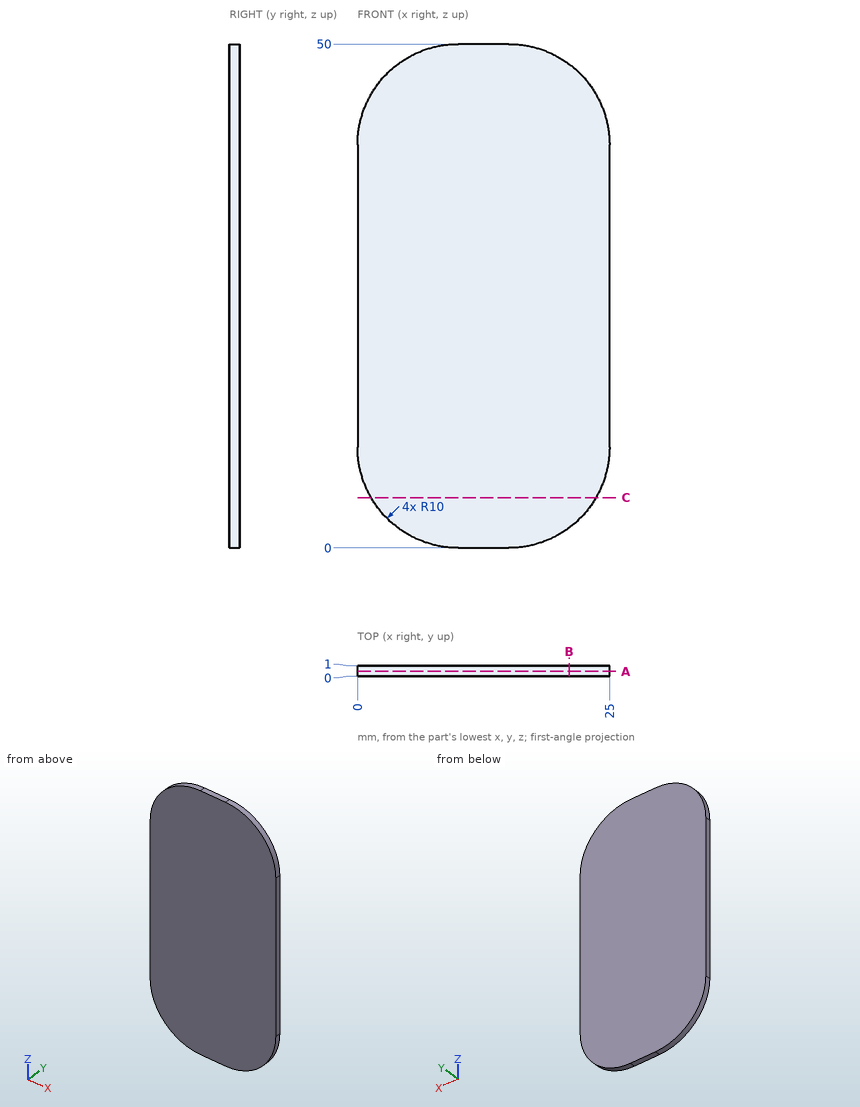
Verification items for this drawing (mm, ordinates from the low corner). Coordinates: 2 decimals unless noted, no trailing zeros. Order: outer loops, then holes, each group sorted by start corner. A loop starts at its lowest first (then second) coordinate and runs counter-clockwise, first axis right, second up. Notation, with made-up numbers: (88.25, 9.5) - (144.25, 9.5) arc R34 cw to (144.25, 43.5) - close; hole circle Ø3 at (63, 32.25). An arc over 180 degrees is marked (long way). Answer in a Markdown table with one row per item. Add a question column.
1. Section check B-B (x = 21). Enter the section's corners in (y, z), plus the area to 3 significant figures.
2. Section check C-C (z = 5). Enter the section's corners in (x, y), plus the area to 3 significant figures.
3. Section check A-A (y = 0.45). Enter the section's corners in (x, z).
4. Material ranges on L1, parallel to Z at x = 15.25, y = 0.65; L2, parallel to Z at x = 21.5, y = 0.45; L3, parallel to X at y = 0.3, z = 9, recorded low to high. Write a range as [from, to].
Data:
| question | item | result |
|---|---|---|
| 1 | outline | (0, 2) - (1, 2) - (1, 48) - (0, 48) - close |
| 1 | area | 46.0 mm² |
| 2 | outline | (1.34, 0) - (23.66, 0) - (23.66, 1) - (1.34, 1) - close |
| 2 | area | 22.3 mm² |
| 3 | outline | (0, 10) arc R10 ccw to (10, 0) - (15, 0) arc R10 ccw to (25, 10) - (25, 40) arc R10 ccw to (15, 50) - (10, 50) arc R10 ccw to (0, 40) - close |
| 4 | L1 | z = [0, 50] |
| 4 | L2 | z = [2.4, 47.6] |
| 4 | L3 | x = [0.05, 24.95] |
